```python
from build123d import *

# Parameters (mm, degrees)
SKETCH_1_W               = 32
SKETCH_1_H               = 34
SKETCH_1_R               = 2.6
EXTRUDE_1_DEPTH          = 2.5
EXTRUDE_START            = -0.5
SKETCH_1_28_W            = 32
SKETCH_1_28_H            = 34
EXTRUDE_2_DEPTH          = 0.5
SKETCH_2_R               = 1.5
CUT_EXTRUDE_1_DEPTH      = 30.983328701
SKETCH_2_3_R             = 2.25
CUT_EXTRUDE_2_DEPTH      = 2.5
SKETCH_3_R               = 0.75
CUT_EXTRUDE_3_DEPTH      = 30.983328701
CUT_EXTRUDE_4_DEPTH      = 30.93743476
CUT_EXTRUDE_4_DEPTH_BACK = 30.93743476
SKETCH_1_29_R            = 1.15


with BuildPart() as part:
    # 草图1 → 凸台-拉伸1 (new body)
    with BuildSketch(Plane(origin=(0, 0, 0), x_dir=(1, 0, 0), z_dir=(0, 1, 0))):
        with Locations((3, 6)):
            Rectangle(SKETCH_1_W, SKETCH_1_H)
        with Locations(Location((0, 0, 0), (0, 0, 270))):
            Circle(SKETCH_1_R, mode=Mode.SUBTRACT)
        with BuildLine():
            ThreePointArc((-1.554347826, 8.564938654), (-6.989130435, 11.48154906), (-1.554347826, 14.398159465))
            ThreePointArc((-1.554347826, 14.398159465), (18.010869565, 11.48154906), (-1.554347826, 8.564938654))
        make_face(mode=Mode.SUBTRACT)
    extrude(amount=EXTRUDE_1_DEPTH)

    # 草图1<28> → 凸台-拉伸2 (add)
    with BuildSketch(Plane(origin=(0, 0, 0), x_dir=(1, 0, 0), z_dir=(0, 1, 0)).offset(EXTRUDE_START)):
        with Locations((3, 6)):
            Rectangle(SKETCH_1_28_W, SKETCH_1_28_H)
        with BuildLine():
            ThreePointArc((-1.554347826, 8.564938654), (-6.989130435, 11.48154906), (-1.554347826, 14.398159465))
            ThreePointArc((-1.554347826, 14.398159465), (18.010869565, 11.48154906), (-1.554347826, 8.564938654))
        make_face(mode=Mode.SUBTRACT)
    extrude(amount=EXTRUDE_2_DEPTH)

    # 草图2 → 切除-拉伸1 (cut, through all)
    with BuildSketch(Plane.XZ.offset(0.5)):
        with Locations(Location((17, -21, 0), (0, 0, 270))):
            Circle(SKETCH_2_R)
        with Locations(Location((-10, 8, 0), (0, 0, 270))):
            Circle(SKETCH_2_R)
        with Locations(Location((16, 8, 0), (0, 0, 270))):
            Circle(SKETCH_2_R)
    extrude(amount=-CUT_EXTRUDE_1_DEPTH, mode=Mode.SUBTRACT)

    # 草图2<3> → 切除-拉伸2 (cut)
    with BuildSketch(Plane.XZ.offset(0.5)):
        with Locations((17, -21)):
            Circle(SKETCH_2_3_R)
        with Locations(Location((-10, 8, 0), (0, 0, 270))):
            Circle(SKETCH_2_3_R)
        with Locations(Location((16, 8, 0), (0, 0, 270))):
            Circle(SKETCH_2_3_R)
    extrude(amount=-CUT_EXTRUDE_2_DEPTH, mode=Mode.SUBTRACT)

    # 草图3 → 切除-拉伸3 (cut, through all)
    with BuildSketch(Plane.XZ.offset(0.5)):
        with Locations(Location((-7, -6, 0), (0, 0, 270))):
            Circle(SKETCH_3_R)
        with Locations(Location((-8, -18, 0), (0, 0, 270))):
            Circle(SKETCH_3_R)
    extrude(amount=-CUT_EXTRUDE_3_DEPTH, mode=Mode.SUBTRACT)

    # 草图1<29> → 切除-拉伸4 (cut, two sides: drawn at the far end of the back side and taken through both)
    with BuildSketch(Plane(origin=(0, 0, 0), x_dir=(1, 0, 0), z_dir=(0, 1, 0)).offset(-CUT_EXTRUDE_4_DEPTH_BACK)):
        with Locations(Location((4.985018819, 0.386765274, 0), (0, 0, 270))):
            Circle(SKETCH_1_29_R)
    extrude(amount=CUT_EXTRUDE_4_DEPTH + CUT_EXTRUDE_4_DEPTH_BACK, mode=Mode.SUBTRACT)


solid = part.part
```
Design review of the part built by this model. Coordinates are the model's own, in mm. A direction names the side the tool comes from. Round coordinates to 2 decimals unless told otherwise and drop trailing zeros. Write each loop counter-clockwise with the first axis right and the second up, starting at its lowest first coordinate (ties: lowest second). Pieces come first, ordered by that corner, then holes. Notation, with made-up numbers: (35, 40) -> (75, 40) arc R27 ccw to (75, 65) -> close; hole circle Ø11 at (35.5, 17.5). An arc over 180 degrees is marked (long way). Answer in a Markdown table with one row per item.
Q1. Draft analysis for pull direction X (two halves, no side actions). For faces 4 (the face through (-10.9, 2.2, 9.2)), 5 (the face through (3, 1, 11)), 6 (the face through (18.01, 2.25, -19.89)), 7 (the face through (19, 1, -6)), state which applies: +X half, -X half, draft (parallel to the pull), parting line (faces both ways), or undercut.
The answers:
| item | result |
|---|---|
| face 4 | undercut |
| face 5 | draft |
| face 6 | undercut |
| face 7 | +X half |
Q2. For faces 1 (the face through (-8.456, 0.979, -17.405)), 2 (the face through (-8.48, 0.73, 9.66)), 3 (the face through (0, 0, 0)), list the 3-axis set-ups (+Z, -Z, +X, -X, +Y, -Y) from which the entire face can be reached by the end or side of a thin tool; tool diameter is ignored.
The answers:
| item | result |
|---|---|
| face 1 | +Y, -Y |
| face 2 | -Y |
| face 3 | +Y |
Q3. Clearance check with flat-ended pins moving along their axes: pin 1 Ø2.5 at (x, z) = (17, -21) entering from +Y; pin 2 Ø4 at (x, z) = (0, 0) entering from +Y; pin 3 Ø2 at (x, z) = (16.5, -20) entering from -Y. State where each tip first meets the part, or that it passes through.
The answers:
| item | result |
|---|---|
| pin 1 | through |
| pin 2 | y = 0 |
| pin 3 | y = 2 |
Q4. To check wall thickness, follow L1, parallel to X at y = 2.35, z = 8; L2, parallel to Z at x = 17, y = 0.65; L3, parallel to X at y = 1.9, z = -1. State the ranges of each line that lie inside material, in increasing order. Write a range as [from, to].
The answers:
| item | result |
|---|---|
| L1 | [-13, -11.5], [-8.5, 14.5], [17.5, 19] |
| L2 | [-18.75, -15.86], [-7.1, 5.98], [10.02, 11] |
| L3 | [-13, -2.4], [2.4, 4.01], [5.96, 19] |
Q5. Take a section at D-D, the plane z = -16. State the section outline as (x, y) points, then the cut area to 3 significant figures.
The answers:
| item | result |
|---|---|
| outline | (-13, -0.5) -> (-0.91, -0.5) -> (-0.91, 2.5) -> (-13, 2.5) -> close; (16.93, -0.5) -> (19, -0.5) -> (19, 2.5) -> (16.93, 2.5) -> close |
| area | 42.5 mm² |
Q6. Take a section at A-A, the plane x = -10. State the section outline as (y, z) points.
The answers:
| item | result |
|---|---|
| outline | (-0.5, -23) -> (2.5, -23) -> (2.5, 6.5) -> (2, 6.5) -> (2, 5.75) -> (-0.5, 5.75) -> close; (-0.5, 10.25) -> (2, 10.25) -> (2, 9.5) -> (2.5, 9.5) -> (2.5, 11) -> (-0.5, 11) -> close |
Q7. Take a section at C-C, the plane y = 1.25. Count the separate pieces of the cut face and the enclosed holes in it, then the cut area to 3 significant figures.
The answers:
| item | result |
|---|---|
| separate pieces | 2 |
| enclosed holes | 7 |
| area | 668 mm² |
Q8. Take a section at B-B, the plane z = 8. State the section outline as (x, y) points.
The answers:
| item | result |
|---|---|
| outline | (-13, -0.5) -> (-12.25, -0.5) -> (-12.25, 2) -> (-11.5, 2) -> (-11.5, 2.5) -> (-13, 2.5) -> close; (-8.5, 2) -> (-7.75, 2) -> (-7.75, -0.5) -> (13.75, -0.5) -> (13.75, 2) -> (14.5, 2) -> (14.5, 2.5) -> (-8.5, 2.5) -> close; (17.5, 2) -> (18.25, 2) -> (18.25, -0.5) -> (19, -0.5) -> (19, 2.5) -> (17.5, 2.5) -> close |
